Verification items for the finished model (mm, model axes). A direction names the side the tool comes from. Give positions to 0.01 mm unless a question says otherwise; leave off trailing zeros. Loops run counter-clockwise (first coordinate to the right, second up) from the corner with the lowest first, then second, coordinate; pieces in that order, holes last. Notation, with made-up numbers: M -15,64 L 9,64 A7 cw 9,68 Z; hole C 63,17 d8. An arc over 180 degrees is marked long. Use a Markdown table: item, result.
from build123d import *

# Parameters (mm, degrees)
SKETCH_1_R               = 21
EXTRUDE_9_DEPTH          = 6
SKETCH_2_R               = 5.15
CUT_EXTRUDE_11_DEPTH     = 3
PATTERN_CIRCULAR_4_COUNT = 8
CUT_EXTRUDE_12_DEPTH     = 1
SKETCH_4_R               = 6.1
CUT_EXTRUDE_13_DEPTH     = 3.5
SKETCH_5_R               = 3.15
SKETCH_5_R_2             = 1.95
CUT_EXTRUDE_14_DEPTH     = 1
SKETCH_6_R               = 4.15
SKETCH_6_R_2             = 3.15
EXTRUDE_10_DEPTH         = 5


with BuildPart() as part:
    # 스케치1 → 보스-돌출9 (new body)
    with BuildSketch(Plane(origin=(0, 0, 0), x_dir=(1, 0, 0), z_dir=(0, 1, 0))):
        Circle(SKETCH_1_R)
    extrude(amount=-EXTRUDE_9_DEPTH)

    # 스케치2 → 컷-돌출11 (cut)
    with BuildSketch(Plane(origin=(0, 0, 0), x_dir=(1, 0, 0), z_dir=(0, 1, 0))):
        with Locations((0, 14.5)):
            Circle(SKETCH_2_R)
    cut_extrude_11 = extrude(amount=-CUT_EXTRUDE_11_DEPTH, mode=Mode.SUBTRACT)

    # 원형 패턴4: 컷-돌출11 ×8 about axis
    pattern_circular_4_axis = Axis((0, 0, 0), (0, 1, 0))
    for i in range(1, PATTERN_CIRCULAR_4_COUNT):
        add(cut_extrude_11.rotate(pattern_circular_4_axis, i * 360 / PATTERN_CIRCULAR_4_COUNT), mode=Mode.SUBTRACT)

    # 스케치3 → 컷-돌출12 (cut)
    with BuildSketch(Plane.XZ.offset(6)):
        Polygon((-14.320132754, -5.931593202), (-5.931593202, -14.320132754), (5.931593202, -14.320132754), (14.320132754, -5.931593202), (14.320132754, 5.931593202), (5.931593202, 14.320132754), (-5.931593202, 14.320132754), (-14.320132754, 5.931593202), align=None)
        Polygon((-5.434536927, -13.120132754), (5.434536927, -13.120132754), (13.120132754, -5.434536927), (13.120132754, 5.434536927), (5.434536927, 13.120132754), (-5.434536927, 13.120132754), (-13.120132754, 5.434536927), (-13.120132754, -5.434536927), align=None, mode=Mode.SUBTRACT)
    extrude(amount=-CUT_EXTRUDE_12_DEPTH, mode=Mode.SUBTRACT)

    # 스케치4 → 컷-돌출13 (cut)
    with BuildSketch(Plane(origin=(0, 0, 0), x_dir=(1, 0, 0), z_dir=(0, 1, 0))):
        Circle(SKETCH_4_R)
    extrude(amount=-CUT_EXTRUDE_13_DEPTH, mode=Mode.SUBTRACT)

    # 스케치5 → 컷-돌출14 (cut)
    with BuildSketch(Plane.XZ.offset(6)):
        Circle(SKETCH_5_R)
        Circle(SKETCH_5_R_2, mode=Mode.SUBTRACT)
    extrude(amount=-CUT_EXTRUDE_14_DEPTH, mode=Mode.SUBTRACT)

    # 스케치6 → 보스-돌출10 (add)
    with BuildSketch(Plane.XZ.offset(6)):
        Circle(SKETCH_6_R)
        Circle(SKETCH_6_R_2, mode=Mode.SUBTRACT)
    extrude(amount=EXTRUDE_10_DEPTH)


solid = part.part
(1) Cross-section at A-A on y = -2. State how many separate pieces and enclosed holes the cut face has, then the cut area to 3 significant figures.
Results below:
| item | result |
|---|---|
| separate pieces | 1 |
| enclosed holes | 9 |
| area | 602 mm^2 |
(2) Set-up check for faces 1 (the flat face through (-9.224, -5.507, 9.331)), 2 (the flat face through (0, -3.5, 0)), 3 (the cylindrical face through (20.03, -2.96, -6.31)): record each of +Z, -Z, +X, -X, +Y, -Y from which the full face is reachable in a straight line by a thin tool's end or side.
Results below:
| item | result |
|---|---|
| face 1 | -Y |
| face 2 | +Y |
| face 3 | +Y, -Y |
(3) Cross-section at D-D on y = -4.5. Record the cut outline in (x, z), then the cut area to 3 significant figures.
Results below:
| item | result |
|---|---|
| outline | C 0,0 d42 |
| area | 1,390 mm^2 |
(4) Cross-section at C-C on z = 11.5. Record the cut outline in (x, y).
Results below:
| item | result |
|---|---|
| outline | M -17.57,-6 L -8.75,-6 L -8.75,-5 L -7.05,-5 L -7.05,-6 L 7.05,-6 L 7.05,-5 L 8.75,-5 L 8.75,-6 L 17.57,-6 L 17.57,0 L 15.25,0 L 15.25,-3 L 5.26,-3 L 5.26,0 L 4.19,0 L 4.19,-3 L -4.19,-3 L -4.19,0 L -5.26,0 L -5.26,-3 L -15.25,-3 L -15.25,0 L -17.57,0 Z |
(5) Gauge pin test, flat ends, axial feed: P1, Ø10, axis at x = 14, z = 4, coming from the -Y side; P2, Ø5, axis at x = -12.5, z = -9.5, coming from the +Y side; P3, Ø0.5, axis at x = 2, y = -5.5, coming from the -Z side. Record the tip position at first contact, or that the pin passes through.
Results below:
| item | result |
|---|---|
| P1 | y = -6 |
| P2 | y = -3 |
| P3 | z = -20.93 |
(6) Draft check along X on faces 4 (the flat face through (10.07, -5.51, -10.18)), 5 (the flat face through (2, -11, 3)), 6 (the cylindrical face through (-0.9, -8.46, -4.05)). Enter one of: +X half, -X half, draft (parallel to the pull), parting line (faces both ways), or undercut.
Results below:
| item | result |
|---|---|
| face 4 | undercut |
| face 5 | draft |
| face 6 | parting line |
(7) Cross-section at B-B on y = -7. Record the cut outline in (x, z), then the cut area to 3 significant figures.
Results below:
| item | result |
|---|---|
| outline | C 0,0 d8.3; hole C 0,0 d6.3 |
| area | 22.9 mm^2 |
(8) Material ranges on line 1 (Z direction, x = 0, y = -1.7); line 2 (X direction, y = -2, z = 11), recorded low to high.
Results below:
| item | result |
|---|---|
| line 1 | -21 to -19.65, -9.35 to -6.1, 6.1 to 9.35, 19.65 to 21 |
| line 2 | -17.89 to -15.35, -5.16 to -3.78, 3.78 to 5.16, 15.35 to 17.89 |
